Source: CAD feature listing. Evaluate the final solid. Frame: model axes, mm. A direction names the side the tool comes from. Give positions to 0.01 mm unless a question says otherwise; leave off trailing zeros. Write each loop counter-clockwise with the first axis right and the second up, starting at its lowest first coordinate (ties: lowest second). Pieces come first, ordered by that corner, then holes.
```python
from build123d import *

# Parameters (mm, degrees)
CROQUIS1_W              = 25.65
CROQUIS1_H              = 17.8
SALIENTE_EXTRUIR1_DEPTH = 2.5
SALIENTE_EXTRUIR2_DEPTH = 2.2
CROQUIS3_R              = 3.1
CORTAR_EXTRUIR1_DEPTH   = 18.8
CORTAR_EXTRUIR2_DEPTH   = 16.1
REDONDEO1_R             = 5


with BuildPart() as part:
    # Croquis1 → Saliente-Extruir1 (new body)
    with BuildSketch(Plane(origin=(0, 0, 0), x_dir=(1, 0, 0), z_dir=(0, 1, 0))):
        Rectangle(CROQUIS1_W, CROQUIS1_H)
    extrude(amount=SALIENTE_EXTRUIR1_DEPTH)

    # Croquis2 → Saliente-Extruir2 (add)
    with BuildSketch(Plane.XY.offset(8.9)):
        Polygon((-25.125, 0), (12.825, 0), (12.825, 7.9), (-1.375, 15.1), (-25.125, 15.1), align=None)
    saliente_extruir2 = extrude(amount=-SALIENTE_EXTRUIR2_DEPTH)

    # Simetría1: Saliente-Extruir2 across plane
    add(saliente_extruir2.mirror(Plane.XY))

    # Croquis3 → Cortar-Extruir1 (cut, through all)
    with BuildSketch(Plane.XY.offset(8.9)):
        with Locations((-18.225, 7.55)):
            Circle(CROQUIS3_R)
    extrude(amount=-CORTAR_EXTRUIR1_DEPTH, mode=Mode.SUBTRACT)

    # Croquis4 → Cortar-Extruir2 (cut, through all)
    with BuildSketch(Plane.XZ):
        with BuildLine():
            Line((-2.175, 1.5), (-2.175, -1.5))
            ThreePointArc((-2.175, -1.5), (-4.175, -3.5), (-6.175, -1.5))
            Line((-6.175, -1.5), (-6.175, 1.5))
            ThreePointArc((-6.175, 1.5), (-4.175, 3.5), (-2.175, 1.5))
        make_face()
        with BuildLine():
            Line((3.025, -1.5), (3.025, 1.5))
            ThreePointArc((3.025, 1.5), (5.025, 3.5), (7.025, 1.5))
            Line((7.025, 1.5), (7.025, -1.5))
            ThreePointArc((7.025, -1.5), (5.025, -3.5), (3.025, -1.5))
        make_face()
    extrude(amount=-CORTAR_EXTRUIR2_DEPTH, mode=Mode.SUBTRACT)

    # Redondeo1
    redondeo1_edges = [part.edges().sort_by_distance(p)[0] for p in [
        (-25.125, 0, 7.8),
        (-25.125, 15.1, 7.8),
        (-25.125, 0, -7.8),
        (-25.125, 15.1, -7.8),
    ]]
    fillet(redondeo1_edges, radius=REDONDEO1_R)


solid = part.part
```
1. Line query: probe 1 along Z at (x, y) = (-1, 5.5); probe 2 along X at (y, z) = (0.75, 2.25) (3 decimals); probe 3 along Y at (x, z) = (4, 3.5). Output: solid intervals per line, ascending.
2. Pull-direction query (X, two-part tool) for faces 4 (the cylindrical face through (-15.361, 6.363, 7.815)), 5 (the flat face through (-11, 15.1, 8)), 6 (the flat face through (-25.125, 8, 8)), 7 (the cylindrical face through (-4.2, 1.2, 3.5)); classes: pulls with the +X half, pulls with the -X half, needs draft (parallel to the pull), parting line crosses it, or undercut.
3. Access query for faces 1 (the flat face through (0, 2.5, 0)), 2 (the flat face through (3.025, 1, 0)), 3 (the flat face through (0, 0, 0)). Directions: +Z, -Z, +X, -X, +Y, -Y. A direction counts if a zero-diameter tool reaches every point of the face in a straight line with its end or side. Return the directions, or none.
4. Section query A-A (z = 1). Return loops of the section in (x, y) (3 decimals).
5. Section query B-B (x = -18). Return loops of the section in (y, z), plus the area to 3 significant figures.
6. Pin query (flat end, axial travel): P1, Ø1.5, axis at x = 9, z = -7, coming from the +Y side; P2, Ø4, axis at x = 4.5, z = -1, coming from the +Y side; P3, Ø1.2, axis at y = 2, z = 3, coming from the -X side (3 decimals). Return the tip coordinate at first contact, or that it passes through.
7. Section query D-D (y = 8.75). Return loops of the section in (x, z) (3 decimals).
8. Section query C-C (y = 4). Return loops of the section in (x, z) (3 decimals).
The answers:
1. probe 1: z = -8.9 to -6.7, 6.7 to 8.9
1. probe 2: x = -12.825 to -6.029, -2.321 to 3.171, 6.879 to 12.825
1. probe 3: y = 0 to 2.5
2. face 4: undercut
2. face 5: needs draft
2. face 6: pulls with the -X half
2. face 7: undercut
3. face 1: +X, -X, +Y
3. face 2: +Y, -Y
3. face 3: +Z, -Z, +X, -X, -Y
4. outline: (-12.825, 0) - (-6.175, 0) - (-6.175, 2.5) - (-12.825, 2.5) - close; (-2.175, 0) - (3.025, 0) - (3.025, 2.5) - (-2.175, 2.5) - close; (7.025, 0) - (12.825, 0) - (12.825, 2.5) - (7.025, 2.5) - close
5. outline: (0, -8.9) - (4.46, -8.9) - (4.46, -6.7) - (0, -6.7) - close; (0, 6.7) - (4.46, 6.7) - (4.46, 8.9) - (0, 8.9) - close; (10.64, -8.9) - (15.1, -8.9) - (15.1, -6.7) - (10.64, -6.7) - close; (10.64, 6.7) - (15.1, 6.7) - (15.1, 8.9) - (10.64, 8.9) - close
5. area: 39.2 mm2
6. P1: stops at y = 10.22
6. P2: stops at y = 2.5
6. P3: stops at x = -12.825
7. outline: (-25.125, -8.9) - (-21.083, -8.9) - (-21.083, -6.7) - (-25.125, -6.7) - close; (-25.125, 6.7) - (-21.083, 6.7) - (-21.083, 8.9) - (-25.125, 8.9) - close; (-15.367, -8.9) - (11.149, -8.9) - (11.149, -6.7) - (-15.367, -6.7) - close; (-15.367, 6.7) - (11.149, 6.7) - (11.149, 8.9) - (-15.367, 8.9) - close
8. outline: (-25.024, -8.9) - (12.825, -8.9) - (12.825, -6.7) - (-25.024, -6.7) - close; (-25.024, 6.7) - (12.825, 6.7) - (12.825, 8.9) - (-25.024, 8.9) - close
